```python
from build123d import *

# Parameters (mm, degrees)
EXTRUDE_1_DEPTH     = 4
SKETCH_3_R          = 9.242846329
CUT_EXTRUDE_2_DEPTH = 8
SKETCH_5_W          = 39
SKETCH_5_H          = 40.905653917
EXTRUDE_2_DEPTH     = 4
EXTRUDE_3_DEPTH     = 4
SKETCH_8_R          = 9.245
CUT_EXTRUDE_3_DEPTH = 4


with BuildPart() as part:
    # 草图2 → 凸台-拉伸1 (new body)
    with BuildSketch(Plane(origin=(0, 0, 0), x_dir=(1, 0, 0), z_dir=(0, 1, 0))):
        with BuildLine():
            Line((-19.5, 0), (-19.5, 180))
            ThreePointArc((-19.5, 180), (0, 199.5), (19.5, 180))
            Line((19.5, 180), (19.5, 0))
            ThreePointArc((19.5, 0), (0, -19.5), (-19.5, 0))
        make_face()
    extrude_1 = extrude(amount=EXTRUDE_1_DEPTH)

    # 草图3 → 切除-拉伸2 (cut)
    with BuildSketch(Plane(origin=(0, 4, 0), x_dir=(-1, 0, 0), z_dir=(0, 1, 0))):
        with Locations(Location((0, -180, 0), (0, 0, 90))):
            Circle(SKETCH_3_R)
        with Locations(Location((0, 0, 0), (0, 0, 90))):
            Circle(SKETCH_3_R)
    cut_extrude_2 = extrude(amount=-CUT_EXTRUDE_2_DEPTH, mode=Mode.SUBTRACT)

    # 草图5 → 凸台-拉伸2 (add)
    with BuildSketch(Plane(origin=(0, 0, 0), x_dir=(1, 0, 0), z_dir=(0, 1, 0))):
        with Locations((0, 73.039937417)):
            Rectangle(SKETCH_5_W, SKETCH_5_H)
    extrude_2 = extrude(amount=-EXTRUDE_2_DEPTH)

    # 镜向3: 凸台-拉伸1, 切除-拉伸2, 凸台-拉伸2 across plane
    add(extrude_1.mirror(Plane(origin=(0, -4, 0), x_dir=(0, 0, 1), z_dir=(0, -1, 0))))
    add(cut_extrude_2.mirror(Plane(origin=(0, -4, 0), x_dir=(0, 0, 1), z_dir=(0, -1, 0))), mode=Mode.SUBTRACT)
    add(extrude_2.mirror(Plane(origin=(0, -4, 0), x_dir=(0, 0, 1), z_dir=(0, -1, 0))))

    # 草图7 → 凸台-拉伸3 (add)
    with BuildSketch(Plane.XZ.offset(12)):
        with BuildLine():
            Line((11.205673107, -163.975801314), (93.155923926, -221.283360943))
            ThreePointArc((93.155923926, -221.283360943), (97.974449505, -248.513232736), (70.744577713, -253.331758315))
            Line((70.744577713, -253.331758315), (-11.205673107, -196.024198686))
            ThreePointArc((-11.205673107, -196.024198686), (-16.024198686, -168.794326893), (11.205673107, -163.975801314))
        make_face()
    extrude_3 = extrude(amount=-EXTRUDE_3_DEPTH)

    # 草图8 → 切除-拉伸3 (cut)
    with BuildSketch(Plane.XZ.offset(12)):
        with Locations(Location((0, -180.667521799, 0), (0, 0, 270))):
            Circle(SKETCH_8_R)
    cut_extrude_3 = extrude(amount=-CUT_EXTRUDE_3_DEPTH, mode=Mode.SUBTRACT)

    # 镜向6: 凸台-拉伸3, 切除-拉伸3 across plane
    add(extrude_3.mirror(Plane(origin=(0, -4, 0), x_dir=(0, 0, 1), z_dir=(0, -1, 0))))
    add(cut_extrude_3.mirror(Plane(origin=(0, -4, 0), x_dir=(0, 0, 1), z_dir=(0, -1, 0))), mode=Mode.SUBTRACT)


solid = part.part
```
Work out the finished part from the listing and answer in its coordinate system (mm). A direction names the side the tool comes from. Give positions to 0.01 mm unless a question says otherwise; leave off trailing zeros. Loops run counter-clockwise (first coordinate to the right, second up) from the corner with the lowest first, then second, coordinate; pieces in that order, holes last. Notation, with made-up numbers: (85, 73) - (130, 73) arc R10 ccw to (130, 82) - close; hole circle Ø11 at (53.25, -4). An arc over 180 degrees is marked (long way). Use CSV: the item, a comma, the result in double quotes. Start each with the question number.
(1) Each of these flat-tipped pins is pushed along its axis until it touches: pin 1 (16.5 mm diameter, centred on x = 0, z = 0, fed in from +Y); pin 2 (2.5 mm diameter, centred on x = 3, y = -3, fed in from -Z); pin 3 (6 mm diameter, centred on y = 1, z = -116, fed in from +X); pin 4 (8 mm diameter, centred on x = 73.5, y = -5, fed in from -Z). Where does it stop, or does it pass through?
(2) A tool of negligible diameter and unlimited length cuts with its end or side. For faces 1 (the face through (0, -8, -25)), 2 (the face through (28, 0, -176)), 3 (the face through (55.812, 2.028, -195.169)), from which of +Z, -Z, +X, -X, +Y, -Y can it reach the whole face along a straight path? Write none if from no direction.
(3) Find section A-A, the plane z = -47.5. Determine the outline of the cut face in (x, y).
(4) Determine the mould class of faces 4 (the face through (19.5, -4, -84)), 5 (the face through (2.776, -10.028, 8.816)), 6 (the face through (30.343, -10.028, -225.079)) for opening direction X: released by +X, released by -X, zero draft, split by the parting line, or undercut.
(5) Find the intervals of material crossed by L1, parallel to X at y = -10.1, z = 0; L2, parallel to Y at x = 68, z = -217.5; L3, parallel to X at y = 3, z = -90, in increasing order.
(6) Find section C-C, the plane x = 0. Determine the outline of the cut face in (y, z), plus the area to 3 significant figures.
(7) Find section D-D, the plane z = -3. Determine the outline of the cut face in (x, y).
(8) Find section B-B, the plane x = 73.5. Determine the outline of the cut face in (y, z).
Results found:
1,pin 1,"through"
1,pin 2,"z = -93.49"
1,pin 3,"x = 19.5"
1,pin 4,"z = -255.98"
2,face 1,"+Z, +X, -X"
2,face 2,"-Z, +X, -X"
2,face 3,"+Z, +X, +Y, -Y"
3,outline,"(-19.5, -12) - (19.5, -12) - (19.5, -8) - (-19.5, -8) - close; (-19.5, 0) - (19.5, 0) - (19.5, 4) - (-19.5, 4) - close"
4,face 4,"released by +X"
4,face 5,"undercut"
4,face 6,"released by -X"
5,L1,"-19.5 to -9.24, 9.24 to 19.5"
5,L2,"-12 to -8, 0 to 4"
5,L3,"-19.5 to 19.5"
6,outline,"(-12, -203.86) - (-8, -203.86) - (-8, -189.91) - (-12, -189.91) - close; (-12, -171.42) - (-8, -171.42) - (-8, -93.49) - (0, -93.49) - (0, -171.42) - (4, -171.42) - (4, -9.24) - (0, -9.24) - (0, -52.59) - (-8, -52.59) - (-8, -9.24) - (-12, -9.24) - close; (-12, 9.24) - (-8, 9.24) - (-8, 19.5) - (-12, 19.5) - close; (0, -203.86) - (4, -203.86) - (4, -189.91) - (0, -189.91) - close; (0, 9.24) - (4, 9.24) - (4, 19.5) - (0, 19.5) - close"
6,area,"1,820 mm^2"
7,outline,"(-19.5, -12) - (-8.74, -12) - (-8.74, -8) - (-19.5, -8) - close; (-19.5, 0) - (-8.74, 0) - (-8.74, 4) - (-19.5, 4) - close; (8.74, -12) - (19.5, -12) - (19.5, -8) - (8.74, -8) - close; (8.74, 0) - (19.5, 0) - (19.5, 4) - (8.74, 4) - close"
8,outline,"(-12, -254.94) - (-8, -254.94) - (-8, -207.54) - (-12, -207.54) - close; (0, -254.94) - (4, -254.94) - (4, -207.54) - (0, -207.54) - close"
